Design review of the part shown in the three views and the two pictorial views. Dimensions are in mm from the part's minimum x, y and z. A direction names the side the tool comes from. Coordinates: 2 decimals unless noted, no trailing zeros. Write each loop counter-clockwise with the first axis right and the second up, starting at its lowest first coordinate (ties: lowest second). Pieces come first, ordered by that corner, then holes. Notation, with made-up numbers: (-39.75, 70) -> (-15.75, 70) arc R16 cw to (-15.75, 91) -> close; hole circle Ø7 at (34.25, 53). An arc over 180 degrees is marked (long way). Answer in a Markdown table with one row per item. Add a question column.
Item 1: Take a section at B-B, the plane y = 55. Write out the cut boundary in (x, z), and give its area (3 significant figures).
Item 2: Take a section at C-C, the plane z = 12. Write out the cut boundary in (x, y), and give its area (3 significant figures).
Item 3: To check wall thickness, follow line 1 (X direction, y = 55, z = 5); line 2 (Z direction, x = 5.5, y = 27); line 3 (Y direction, x = 10, z = 4.5). State the ranges of each line that lie inside material, in increasing order.
Item 4: Clearance check with flat-ended pins moving along their axes: P1, Ø4, axis at x = 5.5, y = 53.5, coming from the -Z side; P2, Ø2, axis at x = 10, y = 5, coming from the +Z side; P3, Ø2, axis at x = 15, y = 29.5, coming from the -Z side. State where each tip first meets the part, or that it passes through.
Item 5: Take a section at A-A, the plane x = 10. Write out the cut boundary in (y, z), and give its area (3 significant figures).
Item 6: Draft analysis for pull direction Z (two halves, no side actions). For the marked faces 4, 5 and 6, state which applies: released by +Z, released by -Z, zero draft, split by the parting line, or undercut.
Item 7: For the marked faces 1, 2 and 3, list the 3-axis set-ups (+Z, -Z, +X, -X, +Y, -Y) from which the entire face can be reached by the end or side of a thin tool; tool diameter is ignored.
Item 8: Take a section at D-D, the plane x = 14.25. Write out the cut boundary in (y, z).
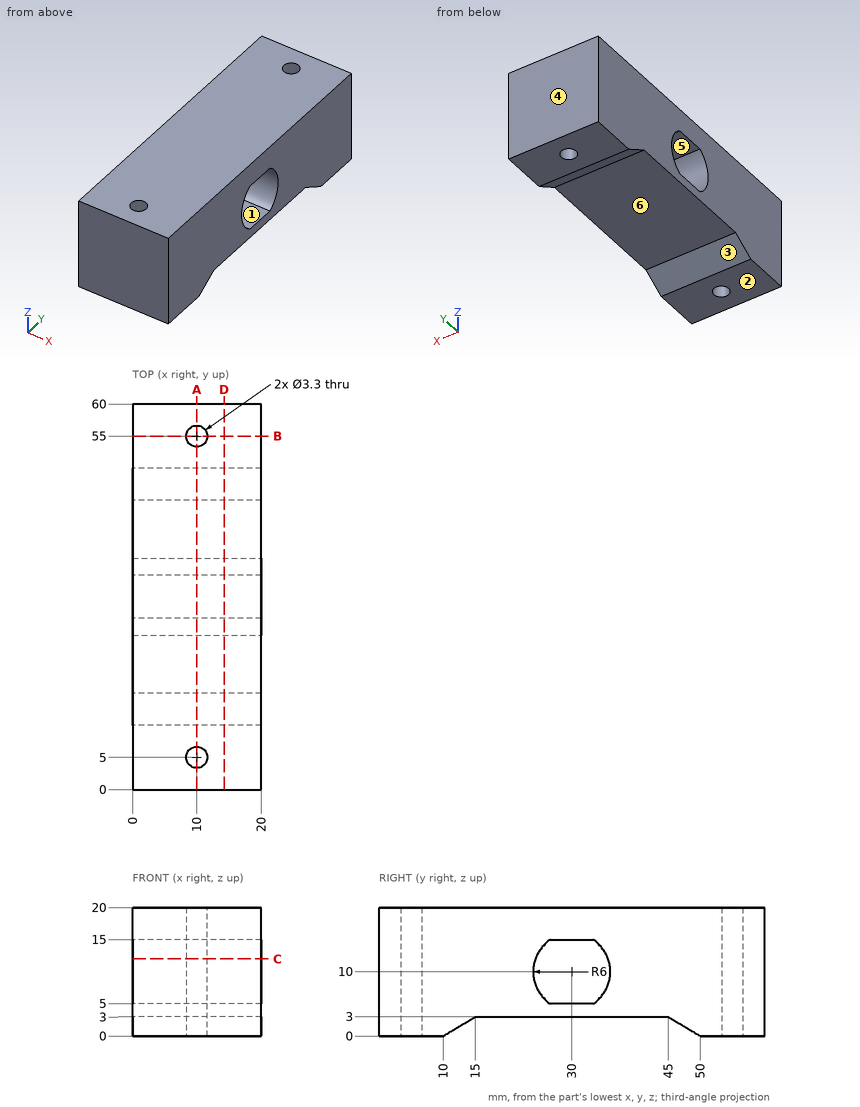
Answers:
| question | item | result |
|---|---|---|
| 1 | outline | (0, 0) -> (8.35, 0) -> (8.35, 20) -> (0, 20) -> close; (11.65, 0) -> (20, 0) -> (20, 20) -> (11.65, 20) -> close |
| 1 | area | 334 mm^2 |
| 2 | outline | (0, 0) -> (20, 0) -> (20, 24.34) -> (0, 24.34) -> close; (0, 35.66) -> (20, 35.66) -> (20, 60) -> (0, 60) -> close; hole circle Ø3.3 at (10, 5); hole circle Ø3.3 at (10, 55) |
| 2 | area | 957 mm^2 |
| 3 | line 1 | x = 0 to 8.35, 11.65 to 20 |
| 3 | line 2 | z = 3 to 5, 15 to 20 |
| 3 | line 3 | y = 0 to 3.35, 6.65 to 53.35, 56.65 to 60 |
| 4 | P1 | stops at z = 0 |
| 4 | P2 | passes through |
| 4 | P3 | stops at z = 3 |
| 5 | outline | (0, 0) -> (3.35, 0) -> (3.35, 20) -> (0, 20) -> close; (6.65, 0) -> (10, 0) -> (15, 3) -> (45, 3) -> (50, 0) -> (53.35, 0) -> (53.35, 20) -> (6.65, 20) -> close; (56.65, 0) -> (60, 0) -> (60, 20) -> (56.65, 20) -> close; hole (26.68, 5) -> (33.32, 5) arc R6 ccw to (33.32, 15) -> (26.68, 15) arc R6 ccw to start |
| 5 | area | 859 mm^2 |
| 6 | face 4 | zero draft |
| 6 | face 5 | undercut |
| 6 | face 6 | released by -Z |
| 7 | face 1 | +X, -X |
| 7 | face 2 | -Z, +X, -X, +Y, -Y |
| 7 | face 3 | -Z, +X, -X |
| 8 | outline | (0, 0) -> (10, 0) -> (15, 3) -> (45, 3) -> (50, 0) -> (60, 0) -> (60, 20) -> (0, 20) -> close; hole (26.68, 5) -> (33.32, 5) arc R6 ccw to (33.32, 15) -> (26.68, 15) arc R6 ccw to start |
